Check sheet for the modelled part. Datum: model origin and axes. Units: mm. A direction names the side the tool comes from. Coordinates: 2 decimals unless noted, no trailing zeros. Write each loop counter-clockwise with the first axis right and the second up, starting at its lowest first coordinate (ties: lowest second). Pieces come first, ordered by that corner, then holes. Notation, with made-up numbers: (-37.5, -21.5) - (-5.5, -21.5) arc R17 ccw to (-5.5, -2.5) - close; hole circle Ø8 at (13, -40). An arc over 180 degrees is marked (long way). Write each question's results on one line, items separated by ' | '.
from build123d import *

# Parameters (mm, degrees)
SKETCH1_W               = 174.879
SKETCH1_H               = 25.4
BOSS_EXTRUDE1_DEPTH     = 3.175
SKETCH2_W               = 22.225
SKETCH2_H               = 3.175
CUT_EXTRUDE1_DEPTH      = 177.742482912
F_1_4_CLEARANCE_HOLE1_D = 6.7564


with BuildPart() as part:
    # Sketch1 → Boss-Extrude1 (new body)
    with BuildSketch(Plane.XY):
        with Locations((-87.4395, -12.7)):
            Rectangle(SKETCH1_W, SKETCH1_H)
    extrude(amount=BOSS_EXTRUDE1_DEPTH)

    # Sketch2 → Cut-Extrude1 (cut, through all)
    with BuildSketch(Plane.XY.offset(3.175)):
        with Locations((-163.7665, -23.8125)):
            Rectangle(SKETCH2_W, SKETCH2_H)
    cut_extrude1 = extrude(amount=-CUT_EXTRUDE1_DEPTH, mode=Mode.SUBTRACT)

    # Mirror1: Cut-Extrude1 across plane
    add(cut_extrude1.mirror(Plane.ZY.offset(87.4395)), mode=Mode.SUBTRACT)

    # 1/4 Clearance Hole1 (through all)
    with Locations(Plane.XY.offset(3.175)):
        with Locations((-46.1645, -15.875), (-128.7145, -15.875)):
            Hole(F_1_4_CLEARANCE_HOLE1_D / 2)


solid = part.part
1. Material ranges on L1, parallel to X at y = -16.25, z = 2.75; L2, parallel to X at y = -15, z = 2.05; L3, parallel to Y at x = -44, z = 2.6, recorded low to high. Write a range as [from, to].
Values follow:
L1: x = [-174.88, -132.07], [-125.36, -49.52], [-42.81, 0] | L2: x = [-174.88, -131.98], [-125.45, -49.43], [-42.9, 0] | L3: y = [-25.4, -18.47], [-13.28, 0]
2. Sectioned sample at B-B (z = 1.25). Record the cut outline in (x, y) (1 decimal), then the cut area to 3 significant figures.
Values follow:
outline: (-174.9, -22.2) - (-152.7, -22.2) - (-152.7, -25.4) - (-22.2, -25.4) - (-22.2, -22.2) - (0, -22.2) - (0, 0) - (-174.9, 0) - close; hole circle Ø6.8 at (-128.7, -15.9); hole circle Ø6.8 at (-46.2, -15.9) | area: 4,230 mm^2
3. Sectioned sample at C-C (x = -13). Record the cut outline in (y, z) (3 decimals), then the cut area to 3 significant figures.
Values follow:
outline: (-22.225, 0) - (0, 0) - (0, 3.175) - (-22.225, 3.175) - close | area: 70.6 mm^2
4. Sectioned sample at A-A (y = -17.75). Record the cut outline in (x, z) (3 decimals), then the cut area to 3 significant figures.
Values follow:
outline: (-174.879, 0) - (-131.525, 0) - (-131.525, 3.175) - (-174.879, 3.175) - close; (-125.904, 0) - (-48.975, 0) - (-48.975, 3.175) - (-125.904, 3.175) - close; (-43.354, 0) - (0, 0) - (0, 3.175) - (-43.354, 3.175) - close | area: 520 mm^2
5. Access from +Z, -Z, +X, -X, +Y, -Y to the whole of each face (thin tool, end or side, straight path). Record for faces 4 (the cylindrical face through (-131.937, -14.86, 1.565)), 5 (the flat face through (-164, -22.225, 2)), 6 (the flat face through (-22.225, -24, 2)).
Values follow:
face 4: +Z, -Z | face 5: +Z, -Z, -X, -Y | face 6: +Z, -Z, +X, -Y
6. Draft check along Y on faces 1 (the flat face through (-152.654, -24, 2)), 2 (the flat face through (-11, -22.225, 2)), 3 (the cylindrical face through (-49.4, -14.9, 1.6)). Enter one of: pulls with the +Y half, pulls with the -Y half, needs draft (parallel to the pull), parting line crosses it, or undercut.
Values follow:
face 1: needs draft | face 2: pulls with the -Y half | face 3: undercut
7. Go/stop test with flat-tipped pins: pin 1 (1.6 mm diameter, centred on x = -169, z = 1.5, fed in from -Y) (3 decimals); pin 2 (1 mm diameter, centred on y = -23.5, z = 1.5, fed in from +X) (3 decimals). Record where each tip stops, or that it passes through.
Values follow:
pin 1: stops at y = -22.225 | pin 2: stops at x = -22.225
